from build123d import *

# Parameters (mm, degrees)
SKETCH1_W                = 12
SKETCH1_H                = 12
BOSS_EXTRUDE1_DEPTH      = 3
SKETCH2_R                = 5.995277692
BOSS_EXTRUDE2_DEPTH      = 5.4
BOSS_EXTRUDE3_DEPTH      = 2
BOSS_EXTRUDE4_DEPTH      = 0.127
BOSS_EXTRUDE4_DEPTH_BACK = 1.27
SKETCH4_W                = 4
SKETCH4_H                = 3


with BuildPart() as part:
    # Sketch1 → Boss-Extrude1 (new body)
    with BuildSketch(Plane(origin=(0, 0, 0), x_dir=(1, 0, 0), z_dir=(0, 1, 0))):
        Rectangle(SKETCH1_W, SKETCH1_H)
    extrude(amount=BOSS_EXTRUDE1_DEPTH)

    # Sketch2 → Boss-Extrude2 (add)
    with BuildSketch(Plane(origin=(0, 3, 0), x_dir=(1, 0, 0), z_dir=(0, 1, 0))):
        with Locations(Location((0, 0, 0), (0, 0, 90))):
            Circle(SKETCH2_R)
    extrude(amount=BOSS_EXTRUDE2_DEPTH)

    # Sketch3 → Boss-Extrude3 (add)
    with BuildSketch(Plane(origin=(6, 0, 0), x_dir=(0, 0, -1), z_dir=(1, 0, 0))):
        with BuildLine():
            Line((-3.983677321, 1.927671256), (-2.644454293, 1.927671256))
            ThreePointArc((-2.644454293, 1.927671256), (-2.332402325, 1.615619288), (-2.644454293, 1.303567321))
            Line((-2.644454293, 1.303567321), (-3.983677321, 1.303567321))
            ThreePointArc((-3.983677321, 1.303567321), (-4.295729288, 1.615619288), (-3.983677321, 1.927671256))
        make_face()
        with BuildLine():
            Line((3.983677321, 1.927671256), (2.644454293, 1.927671256))
            ThreePointArc((2.644454293, 1.927671256), (2.332402325, 1.615619288), (2.644454293, 1.303567321))
            Line((2.644454293, 1.303567321), (3.983677321, 1.303567321))
            ThreePointArc((3.983677321, 1.303567321), (4.295729288, 1.615619288), (3.983677321, 1.927671256))
        make_face()
    extrude(amount=BOSS_EXTRUDE3_DEPTH)

    # Sketch4 → Boss-Extrude4 (add, two sides: drawn at the far end of the back side and taken through both)
    with BuildSketch(Plane.XZ.offset(-BOSS_EXTRUDE4_DEPTH_BACK)):
        with Locations((0, 4.754)):
            Rectangle(SKETCH4_W, SKETCH4_H)
        with Locations((0, -4.754)):
            Rectangle(SKETCH4_W, SKETCH4_H)
    extrude(amount=BOSS_EXTRUDE4_DEPTH + BOSS_EXTRUDE4_DEPTH_BACK)


solid = part.part
Read the model definition and answer for the solid it produces. Units are mm, in the model's axes. A direction names the side the tool comes from. Round coordinates to 2 decimals unless told otherwise and drop trailing zeros. Write each loop counter-clockwise with the first axis right and the second up, starting at its lowest first coordinate (ties: lowest second). Pieces come first, ordered by that corner, then holes. Notation, with made-up numbers: (-30, 13.25) - (-7, 13.25) arc R15 ccw to (-7, 41.25) - close; hole circle Ø10 at (-14, 6.5). An arc over 180 degrees is marked (long way). Use a Markdown table: item, result.
(1) Which of the six approach directions +Z, -Z, +X, -X, +Y, -Y give full straight-line access (tool end or side, diameter ignored) to faces 1 (the flat face through (7, 1.928, -3)), 2 (the flat face through (7, 1.304, 3)), 3 (the cylindrical face through (-1.8, 5.66, -5.72)), 4 (the flat face through (0, 1, -6.254))?
Reported:
| item | result |
|---|---|
| face 1 | +Z, -Z, +X, +Y |
| face 2 | +Z, -Z, +X, -Y |
| face 3 | +Y |
| face 4 | -Z, +X, -X, +Y, -Y |
(2) Each of these flat-tipped pins is pushed along its axis until it touches: pin 1 Ø1.5 at (y, z) = (0.5, -5) entering from +X; pin 2 Ø3 at (x, y) = (0.5, 6) entering from -Z; pin 3 Ø1.1 at (x, z) = (7.5, 3.5) entering from +Y. Where does it stop, or does it pass through?
Reported:
| item | result |
|---|---|
| pin 1 | x = 6 |
| pin 2 | z = -6 |
| pin 3 | y = 1.93 |
(3) Straight lines are drawn through the part: line 1 along Y through (x, z) = (3.75, 2.5); line 2 along Y through (x, z) = (-5.25, 5.5); line 3 along Z through (x, y) = (0.5, 1.5). For each, find the intervals that lie inside material, in ascending order. Write a range as [from, to].
Reported:
| item | result |
|---|---|
| line 1 | [0, 8.4] |
| line 2 | [0, 3] |
| line 3 | [-6, 6] |
(4) The part is cut by section C-C (y = 7.5). Write down the section's boundary in (x, z), then the cut area to 3 significant figures.
Reported:
| item | result |
|---|---|
| outline | circle Ø11.99 at (0, 0) |
| area | 113 mm2 |
(5) The part is cut by section D-D (z = -1.75). Write down the section's boundary in (x, y), then the cut area to 3 significant figures.
Reported:
| item | result |
|---|---|
| outline | (-6, 0) - (6, 0) - (6, 3) - (5.73, 3) - (5.73, 8.4) - (-5.73, 8.4) - (-5.73, 3) - (-6, 3) - close |
| area | 97.9 mm2 |
